Input: part model. Units: mm. Frame: model coordinates. Face numbers are marked on the shaded views. A direction names the side the tool comes from. Coordinates: 2 decimals unless noted, no trailing zeros. Write each loop counter-clockwise with the first axis right and the second up, starting at its lowest first coordinate (ties: lowest second). Pieces come first, ordered by that corner, then holes. Notation, with made-up numbers: (81, 28) - (119, 28) arc R26 ccw to (119, 61) - close; hole circle Ø5 at (7.25, 37). An arc over 180 degrees is marked (long way). Use a Markdown table: item, result. Add a question column.
Q1. Section query A-A (x = 28.6). Return the cut outline in (y, z), then the cut area to 3 significant figures.
Q2. Section query B-B (z = 5.05). Return the cut outline in (x, y) (3 decimals).
Q3. Mould query, pull axis Y, two halves, no side actions, for the marked faces 4, 5, 6 and 7. Classes: released by +Y, released by -Y, zero draft, split by the parting line, or undercut.
Q4. Set-up query: the marked faces 1, 2 and 3. Return all of +Z, -Z, +X, -X, +Y, -Y with unobstructed straight access to the full face (end or side cutting, diameter ignored); none if empty.
Q5. Section query C-C (z = 9.25). Return the cut outline in (x, y), then the cut area to 3 significant figures.
Q6. Section query D-D (y = 4.5). Return the cut outline in (x, z) (3 decimals).
Q7. Pin query (flat end, axial travel): P1, Ø6, axis at x = 28.6, y = 14.287, coming from the +Z side; P2, Ø2.5, axis at y = 8.5, z = 4, coming from the +X side; P3, Ø1.5, axis at y = 23.5, z = 6, coming from the +X side; P4, Ø2, axis at x = 38.5, z = 8.5, coming from the +Y side. Return the tip coordinate at first contact, or that it passes through.
Q8. Material intervals for probe 1 along Y at (x, z) = (28.5, 0.75); probe 2 along Y at (x, z) = (45, 3); probe 3 along X at (y, z) = (14.75, 3.5), sorted ascending. Write a range as from..to.
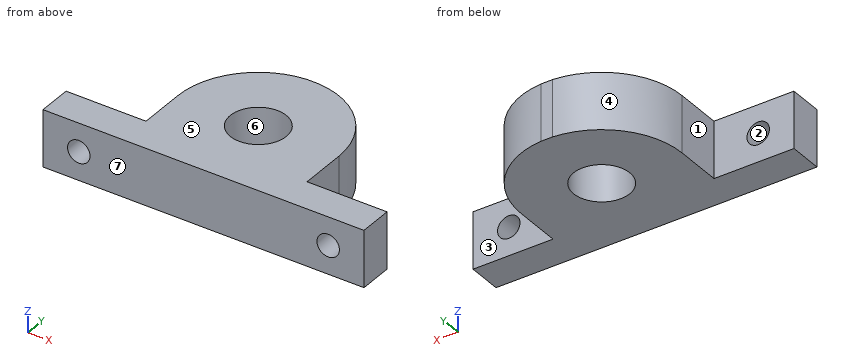
from build123d import *

# Parameters (mm, degrees)
SKETCH1_W               = 57.2
SKETCH1_H               = 28.6
BOSS_EXTRUDE1_DEPTH     = 10.1
SKETCH3_R               = 5
CUT_EXTRUDE2_DEPTH      = 11.1
CUT_EXTRUDE3_DEPTH      = 1
CUT_EXTRUDE3_DEPTH_BACK = 11.1
SKETCH5_R               = 2
CUT_EXTRUDE4_DEPTH      = 6.999141562


with BuildPart() as part:
    # Sketch1 → Boss-Extrude1 (new body)
    with BuildSketch(Plane.XY):
        with Locations((28.6, 14.3)):
            Rectangle(SKETCH1_W, SKETCH1_H)
    extrude(amount=BOSS_EXTRUDE1_DEPTH)

    # Sketch3 → Cut-Extrude2 (cut, through all)
    with BuildSketch(Plane.XY.offset(10.1)):
        with Locations((28.6, 14.287)):
            Circle(SKETCH3_R)
    extrude(amount=-CUT_EXTRUDE2_DEPTH, mode=Mode.SUBTRACT)

    # Sketch4 → Cut-Extrude3 (cut, two sides)
    with BuildSketch(Plane.XY.offset(10.1)) as cut_extrude3_sk:
        with BuildLine():
            Line((-133.041822115, 5.999141562), (0, 5.999141562))
            Line((0, 5.999141562), (14.25, 5.999141562))
            Line((14.25, 5.999141562), (14.25, 14.287))
            ThreePointArc((14.25, 14.287), (28.6, 28.637), (42.95, 14.287))
            Line((42.95, 14.287), (42.95, 5.999141562))
            Line((42.95, 5.999141562), (57.219085061, 5.999141562))
            Line((57.219085061, 5.999141562), (190.260907176, 5.999141562))
            Line((190.260907176, 5.999141562), (190.260907176, 272.082785792))
            Line((190.260907176, 272.082785792), (-133.041822115, 272.082785792))
            Line((-133.041822115, 272.082785792), (-133.041822115, 5.999141562))
        make_face()
    extrude(amount=CUT_EXTRUDE3_DEPTH, mode=Mode.SUBTRACT)
    extrude(cut_extrude3_sk.sketch, amount=-CUT_EXTRUDE3_DEPTH_BACK, mode=Mode.SUBTRACT)

    # Sketch5 → Cut-Extrude4 (cut, through all)
    with BuildSketch(Plane(origin=(0, 5.999141562, 0), x_dir=(-1, 0, 0), z_dir=(0, 1, 0))):
        with Locations((-6.375, 5.05)):
            Circle(SKETCH5_R)
        with Locations((-50.825, 5.05)):
            Circle(SKETCH5_R)
    extrude(amount=-CUT_EXTRUDE4_DEPTH, mode=Mode.SUBTRACT)


solid = part.part
Values follow:
| question | item | result |
|---|---|---|
| 1 | outline | (0, 0) - (9.29, 0) - (9.29, 10.1) - (0, 10.1) - close; (19.29, 0) - (28.6, 0) - (28.6, 10.1) - (19.29, 10.1) - close |
| 1 | area | 188 mm2 |
| 2 | outline | (0, 0) - (4.375, 0) - (4.375, 5.999) - (0, 5.999) - close; (8.375, 0) - (48.825, 0) - (48.825, 5.999) - (42.95, 5.999) - (42.95, 14.287) arc R14.35 ccw to (29.63, 28.6) - (27.57, 28.6) arc R14.35 ccw to (14.25, 14.287) - (14.25, 5.999) - (8.375, 5.999) - close; (52.825, 0) - (57.2, 0) - (57.2, 5.999) - (52.825, 5.999) - close; hole circle Ø10 at (28.6, 14.287) |
| 3 | face 4 | released by +Y |
| 3 | face 5 | zero draft |
| 3 | face 6 | undercut |
| 3 | face 7 | released by -Y |
| 4 | face 1 | +Z, -Z, -X, +Y |
| 4 | face 2 | +Y, -Y |
| 4 | face 3 | +Z, -Z, +X, +Y |
| 5 | outline | (0, 0) - (57.2, 0) - (57.2, 6) - (42.95, 6) - (42.95, 14.29) arc R14.35 ccw to (29.63, 28.6) - (27.57, 28.6) arc R14.35 ccw to (14.25, 14.29) - (14.25, 6) - (0, 6) - close; hole circle Ø10 at (28.6, 14.29) |
| 5 | area | 826 mm2 |
| 6 | outline | (0, 0) - (57.2, 0) - (57.2, 10.1) - (0, 10.1) - close; hole circle Ø4 at (6.375, 5.05); hole circle Ø4 at (50.825, 5.05) |
| 7 | P1 | through |
| 7 | P2 | x = 42.95 |
| 7 | P3 | x = 40.19 |
| 7 | P4 | y = 25.54 |
| 8 | probe 1 | 0..9.29, 19.29..28.6 |
| 8 | probe 2 | 0..6 |
| 8 | probe 3 | 14.26..23.62, 33.58..42.94 |
